Design review of the part shown in the three views and the two pictorial views. Dimensions are in mm from the part's minimum x, y and z. A direction names the side the tool comes from. Give positions to 0.01 mm unless a question says otherwise; leave off trailing zeros. Loops run counter-clockwise (first coordinate to the right, second up) from the corner with the lowest first, then second, coordinate; pieces in that order, holes last. Notation, with made-up numbers: (30, 84.25) -> (60, 84.25) arc R11 ccw to (60, 93.25) -> close; hole circle Ø9 at (20, 22.25). An arc over 180 degrees is marked (long way). Answer as CSV lines item,"result".
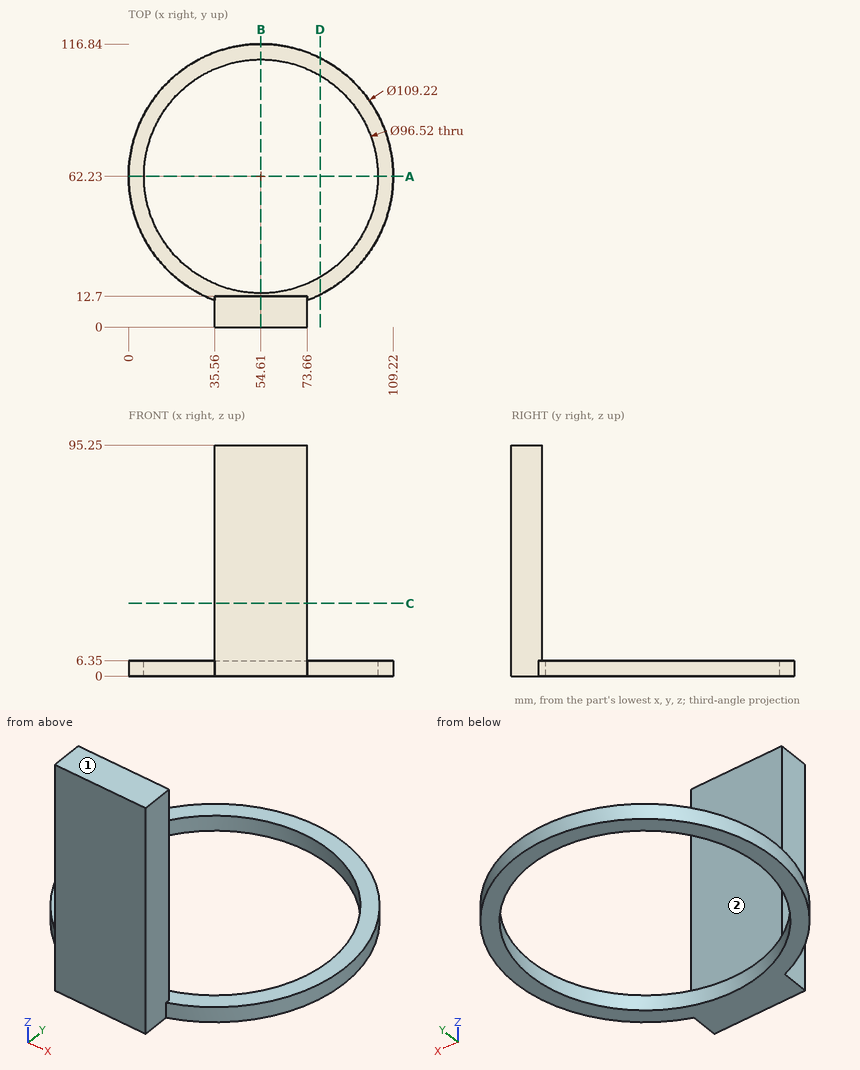
Q1. We need section C-C, the plane z = 30. State the section outline as (x, y) points.
Filled sheet:
outline,"(35.56, 0) -> (73.66, 0) -> (73.66, 12.7) -> (35.56, 12.7) -> close"
Q2. To check wall thickness, follow probe 1 along X at (y, z) = (62, 3); probe 2 along Y at (x, z) = (54.61, 1.75); probe 3 along Y at (x, z) = (42.5, 44). State the ranges of each line that lie inside material, in increasing order. Write a range as from..to.
Filled sheet:
probe 1,"x = 0..6.35, 102.87..109.22"
probe 2,"y = 0..13.97, 110.49..116.84"
probe 3,"y = 0..12.7"
Q3. Clearance check with flat-ended pins moving along their axes: pin 1 Ø19 at (x, z) = (54, 33.5) entering from +Y; pin 2 Ø1.5 at (x, y) = (95, 26) entering from +Z; pin 3 Ø4 at (y, z) = (3.5, 32) entering from -X. State where each tip first meets the part, or that it passes through.
Filled sheet:
pin 1,"stops at y = 12.7"
pin 2,"stops at z = 6.35"
pin 3,"stops at x = 35.56"
Q4. We need section A-A, the plane y = 62.23. State the section outline as (x, z) points, and give its area (3 significant figures).
Filled sheet:
outline,"(0, 0) -> (6.35, 0) -> (6.35, 6.35) -> (0, 6.35) -> close; (102.87, 0) -> (109.22, 0) -> (109.22, 6.35) -> (102.87, 6.35) -> close"
area,"80.6 mm^2"
Q5. We need section D-D, the plane x = 79. State the section outline as (y, z) points.
Filled sheet:
outline,"(13.37, 0) -> (20.59, 0) -> (20.59, 6.35) -> (13.37, 6.35) -> close; (103.87, 0) -> (111.09, 0) -> (111.09, 6.35) -> (103.87, 6.35) -> close"
Q6. For the marked faces 1 and 2, list the 3-axis set-ups (+Z, -Z, +X, -X, +Y, -Y) from which the entire face can be reached by the end or side of a thin tool; tool diameter is ignored.
Filled sheet:
face 1,"+Z, +X, -X, +Y, -Y"
face 2,"+Z, +X, -X, +Y"
Q7. We need section B-B, the plane x = 54.61. State the section outline as (y, z) points, and give its area (3 significant figures).
Filled sheet:
outline,"(0, 0) -> (13.97, 0) -> (13.97, 6.35) -> (12.7, 6.35) -> (12.7, 95.25) -> (0, 95.25) -> close; (110.49, 0) -> (116.84, 0) -> (116.84, 6.35) -> (110.49, 6.35) -> close"
area,"1,260 mm^2"
